Geometry check sheet. Reference: drawing and pictorial views, mm from the part's lowest x, y, z. A direction names the side the tool comes from. Give positions to 0.01 mm unless a question says otherwise; leave off trailing zeros. Order: outer loops, then holes, each group sorted by start corner. A loop starts at its lowest first (then second) coordinate and runs counter-clockwise, first axis right, second up.
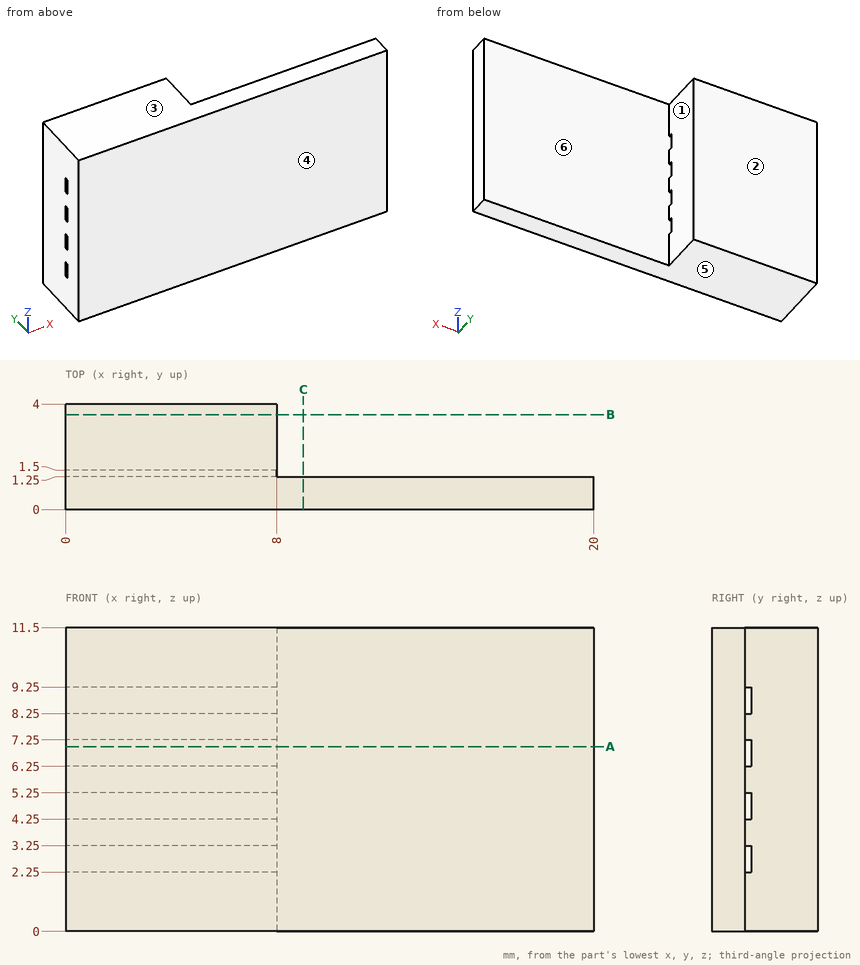
(1) Material ranges on L1, parallel to Y at x = 2, z = 6.75; L2, parallel to Y at x = 17, z = 7.25; L3, parallel to X at y = 1.4, z = 5.75, recorded low to high.
Response values:
L1: y = 0 to 1.25, 1.5 to 4
L2: y = 0 to 1.25
L3: x = 0 to 8
(2) Cross-section at C-C on x = 9. Enter the section's corners in (y, z), then the cut area to 3 significant figures.
Response values:
outline: (0, 0) - (1.25, 0) - (1.25, 11.5) - (0, 11.5) - close
area: 14.4 mm2
(3) Cross-section at B-B on y = 3.6. Enter the section's corners in (x, z), then the cut area to 3 significant figures.
Response values:
outline: (0, 0) - (8, 0) - (8, 11.5) - (0, 11.5) - close
area: 92.0 mm2
(4) Release check for a two-part mould opening along Z. For the marked faces 3, 4, 5 and 6 record: released by +Z, released by -Z, zero draft, split by the parting line, or undercut.
Response values:
face 3: released by +Z
face 4: zero draft
face 5: released by -Z
face 6: undercut
(5) Cross-section at A-A on z = 7. Enter the section's corners in (x, y), then the cut area to 3 significant figures.
Response values:
outline: (0, 0) - (20, 0) - (20, 1.25) - (0, 1.25) - close; (0, 1.5) - (8, 1.5) - (8, 4) - (0, 4) - close
area: 45.0 mm2
(6) Set-up check for the marked faces 1 and 2: record each of +Z, -Z, +X, -X, +Y, -Y from which the full face is reachable in a straight line by a thin tool's end or side.
Response values:
face 1: +Z, -Z, +X, +Y
face 2: +Z, -Z, +X, -X, +Y
